Model file for the job. Use its own axes, mm. A direction names the side the tool comes from. Give positions to 0.01 mm unless a question says otherwise; leave off trailing zeros. Loops run counter-clockwise (first coordinate to the right, second up) from the corner with the lowest first, then second, coordinate; pieces in that order, holes last. Notation, with made-up numbers: M 17.25,63.25 L 43.25,63.25 A17 ccw 43.25,91.25 Z; hole C 54.25,-37 d7. An arc over 180 degrees is marked long. Answer in a Markdown table with one row per item.
```python
from build123d import *

# Parameters (mm, degrees)
SKETCH2_R           = 49.784
BOSS_EXTRUDE1_DEPTH = 203.2
SKETCH3_R           = 11.74839717
BOSS_EXTRUDE2_DEPTH = 50.8


with BuildPart() as part:
    # Sketch1 → Revolve1 (revolve)
    with BuildSketch(Plane.XY):
        with BuildLine():
            Line((304.8, 49.784), (304.8, 0))
            Line((304.8, 0), (0, 0))
            Line((0, 0), (0, 11.748397173))
            add(Edge.make_bspline(
                [(0, 11.748397173), (0.424160675, 11.855932678), (1.277768006, 12.07173392), (3.085410505, 12.527272667), (5.106222596, 13.032281093), (7.110128552, 13.529344024), (9.159948224, 14.034387922), (11.195444228, 14.532141119), (13.233412884, 15.026861964), (15.805049223, 15.64653599), (18.91026091, 16.387291474), (22.550652523, 17.244690048), (26.727238439, 18.213147263), (31.952168035, 19.405675489), (42.412897925, 21.742539102), (62.333903875, 25.976370199), (110.770450737, 35.225121195), (160.70732909, 42.159920913), (207.702302928, 46.434962608), (245.168015054, 48.368183749), (253.734807707, 48.740972714), (260.161369668, 48.98354131), (264.446272339, 49.130442523), (268.731666265, 49.262530797), (273.017475857, 49.379804553), (277.303691578, 49.48226239), (281.590188304, 49.569903083), (285.329649653, 49.633426545), (288.521672796, 49.67849525), (291.166731437, 49.70980578), (293.263778354, 49.731088433), (295.359186858, 49.74882407), (297.470177021, 49.76301264), (299.535126271, 49.773654103), (301.617177871, 49.780748429), (303.482211221, 49.783408805), (304.362420109, 49.784), (304.8, 49.784)],
                knots=[0.082917815, 0.082917815, 0.082917815, 0.082917815, 0.082917815, 0.088601511, 0.094285207, 0.099968902, 0.105652598, 0.111336294, 0.11701999, 0.122703686, 0.128387381, 0.140005218, 0.151623054, 0.16324089, 0.174858727, 0.198094396, 0.267801409, 0.383979763, 0.709279153, 0.744132659, 0.778986165, 0.790604, 0.802221836, 0.813839671, 0.825457507, 0.837075342, 0.848693177, 0.860311013, 0.871928848, 0.877612544, 0.883296239, 0.888979935, 0.89466363, 0.900347326, 0.906031021, 0.911714717, 0.917398412, 0.917398412, 0.917398412, 0.917398412, 0.917398412], degree=4))
        make_face()
    revolve(axis=Axis((304.8, 0, 0), (-1, 0, 0)))

    # Sketch2 → Boss-Extrude1 (add)
    with BuildSketch(Plane(origin=(304.8, 0, 0), x_dir=(0, 0, -1), z_dir=(1, 0, 0))):
        Circle(SKETCH2_R)
    extrude(amount=BOSS_EXTRUDE1_DEPTH)

    # Sketch3 → Boss-Extrude2 (add)
    with BuildSketch(Plane.ZY):
        Circle(SKETCH3_R)
    extrude(amount=BOSS_EXTRUDE2_DEPTH)


solid = part.part
```
Q1. Saw through at B-B (x = 377). Give the cut face in (y, z).
Reported:
| item | result |
|---|---|
| outline | C 0,0 d99.57 |
Q2. Saw through at A-A (x = -8.5). Give the cut face in (y, z), and give its area (3 significant figures).
Reported:
| item | result |
|---|---|
| outline | C 0,0 d23.5 |
| area | 434 mm² |
Q3. Probe probe 1 along Y at (x, z) = (283, -31); probe 2 along Y at (x, z) = (29, 8.5); probe 3 along Z at (x, y) = (208, 41). List the from-to ranges inside material, lowest first.
Reported:
| item | result |
|---|---|
| probe 1 | -38.71 to 38.71 |
| probe 2 | -16.69 to 16.69 |
| probe 3 | -20.86 to 20.86 |
Q4. Drop flat-ended pins along their axis: pin 1 (2 mm diameter, centred on x = 373.5, z = -23, fed in from -Y); pin 2 (8 mm diameter, centred on x = 56, y = -17.5, fed in from -Z); pin 3 (4 mm diameter, centred on x = 147.5, z = 1, fed in from +Y). Give the stop position or say it passes through.
Reported:
| item | result |
|---|---|
| pin 1 | y = -44.66 |
| pin 2 | z = -20.71 |
| pin 3 | y = 40.01 |
Q5. 3-axis set-ups, long thin cutter, end or side, ignore diameter. For faces 1 (the face through (-25.04, 11.65, -1.53)), 2 (the face through (405, -48.6, 10.8)): which of +Z, -Z, +X, -X, +Y, -Y reach the whole face in a straight line?
Reported:
| item | result |
|---|---|
| face 1 | -X |
| face 2 | +X, -X |
